Work out the finished part from the listing and answer in its coordinate system (mm). Give positions to 0.01 mm unless a question says otherwise; leave off trailing zeros. Loops run counter-clockwise (first coordinate to the right, second up) from the corner with the lowest first, then second, coordinate; pieces in that order, holes last. Notation, with made-up numbers: (24.25, 69.25) -> (48.25, 69.25) arc R28 ccw to (48.25, 95.25) -> close; hole circle Ø10 at (15, 78.25). An arc over 180 degrees is marked (long way). Answer as CSV lines item,"result". Start each with the question number.
1. Find the intervals of material crossed by line 1 along X through (y, z) = (70, 4.1); line 2 along X through (y, z) = (78, 1.3); line 3 along X through (y, z) = (6.5, 4.7), in increasing order.
2. Find section C-C, the plane x = 34. Give the vertices of the cut face in (y, z).
3. Determine the mould class of faces 1 (the face through (44.4, 87.7, 2.2)), 2 (the face through (77.5, 45, 3)), 3 (the face through (7.21, 9.73, 2.53)) for opening direction Y: +Y half, -Y half, draft (parallel to the pull), parting line (faces both ways), or undercut.
4. Find section D-D, the plane y = 51.5. Give the vertices of the cut face in (x, z), and give its area (3 significant figures).
5. Find section A-A, the plane x = 7.5. Give the vertices of the cut face in (y, z).
6. Flat-ended cylindrical pins translate along their axes: pin 1 Ø2 at (x, z) = (55, 2) entering from +Y; pin 2 Ø3 at (x, y) = (75, 12) entering from +Z; pin 3 Ø0.6 at (x, z) = (30, 1.5) entering from -Y. Find the tip coordinate at first contact, or state that the pin passes through.
7. Find section B-B, the plane y = 82.5. Give the vertices of the cut face in (x, z), and give its area (3 significant figures).
from build123d import *

# Parameters (mm, degrees)
SKETCH_W        = 90
SKETCH_H        = 90
PAD_DEPTH       = 5
SKETCH001_R     = 2.25
POCKET_DEPTH    = 5
SKETCH002_W     = 65
SKETCH002_H     = 71
POCKET001_DEPTH = 2
SKETCH003_R     = 0.9
POCKET002_DEPTH = 5
SKETCH004_W     = 65
SKETCH004_H     = 60
POCKET003_DEPTH = 3
CHAMFER_SIZE    = 4.5
CHAMFER001_SIZE = 1
CHAMFER002_SIZE = 0.5
CHAMFER003_SIZE = 0.5
CHAMFER004_SIZE = 0.5
CHAMFER005_SIZE = 0.5
CHAMFER006_SIZE = 1
CHAMFER007_SIZE = 0.5
CHAMFER008_SIZE = 0.5
CHAMFER009_SIZE = 0.4
CHAMFER010_SIZE = 0.5


with BuildPart() as part:
    # Sketch → Pad (new body)
    with BuildSketch(Plane.XY):
        with Locations((45, 45)):
            Rectangle(SKETCH_W, SKETCH_H)
    extrude(amount=PAD_DEPTH)

    # Sketch001 (on Face6 of Pad) → Pocket (cut)
    with BuildSketch(Plane.XY.offset(5)):
        with Locations((7.5, 82.5)):
            Circle(SKETCH001_R)
        with Locations((82.5, 82.5)):
            Circle(SKETCH001_R)
        with Locations((82.5, 7.5)):
            Circle(SKETCH001_R)
        with Locations((7.5, 7.5)):
            Circle(SKETCH001_R)
    extrude(amount=-POCKET_DEPTH, mode=Mode.SUBTRACT)

    # Sketch002 (on Face5 of Pocket) → Pocket001 (cut)
    with BuildSketch(Plane.XY.offset(5)):
        with Locations((45, 45)):
            Rectangle(SKETCH002_W, SKETCH002_H)
    extrude(amount=-POCKET001_DEPTH, mode=Mode.SUBTRACT)

    # Sketch003 (on Face15 of Pocket001) → Pocket002 (cut)
    with BuildSketch(Plane.XY.offset(3)):
        with Locations((15, 78)):
            Circle(SKETCH003_R)
        with Locations((41, 78)):
            Circle(SKETCH003_R)
        with Locations((41, 12)):
            Circle(SKETCH003_R)
        with Locations((15, 12)):
            Circle(SKETCH003_R)
        with Locations((49, 78)):
            Circle(SKETCH003_R)
        with Locations((75, 78)):
            Circle(SKETCH003_R)
        with Locations((75, 12)):
            Circle(SKETCH003_R)
        with Locations((49, 12)):
            Circle(SKETCH003_R)
    extrude(amount=-POCKET002_DEPTH, mode=Mode.SUBTRACT)

    # Sketch004 (on Face23 of Pocket002) → Pocket003 (cut)
    with BuildSketch(Plane.XY.offset(3)):
        with Locations((45, 45)):
            Rectangle(SKETCH004_W, SKETCH004_H)
    extrude(amount=-POCKET003_DEPTH, mode=Mode.SUBTRACT)

    # Chamfer
    chamfer_edges = [part.edges().sort_by_distance(p)[0] for p in [
        (45, 90, 0),
        (45, 0, 0),
    ]]
    chamfer(chamfer_edges, length=CHAMFER_SIZE)

    # Chamfer001
    chamfer001_edges = [part.edges().sort_by_distance(p)[0] for p in [
        (0, 45, 0),
        (90, 45, 0),
    ]]
    chamfer(chamfer001_edges, length=CHAMFER001_SIZE)

    # Chamfer002
    chamfer002_edges = [part.edges().sort_by_distance(p)[0] for p in [
        (45, 75, 0),
        (12.5, 45, 0),
        (45, 15, 0),
        (77.5, 45, 0),
    ]]
    chamfer(chamfer002_edges, length=CHAMFER002_SIZE)

    # Chamfer003
    chamfer003_edges = [part.edges().sort_by_distance(p)[0] for p in [
        (5.25, 7.5, 0),
        (80.25, 82.5, 0),
        (80.25, 7.5, 0),
        (5.25, 82.5, 0),
    ]]
    chamfer(chamfer003_edges, length=CHAMFER003_SIZE)

    # Chamfer004
    chamfer004_edges = [part.edges().sort_by_distance(p)[0] for p in [
        (14.1, 78, 0),
        (14.1, 12, 0),
        (40.1, 78, 0),
        (48.1, 12, 0),
        (40.1, 12, 0),
        (48.1, 78, 0),
        (74.1, 12, 0),
        (74.1, 78, 0),
    ]]
    chamfer(chamfer004_edges, length=CHAMFER004_SIZE)

    # Chamfer005
    chamfer005_edges = [part.edges().sort_by_distance(p)[0] for p in [
        (5.25, 7.5, 5),
        (80.25, 7.5, 5),
        (80.25, 82.5, 5),
        (5.25, 82.5, 5),
    ]]
    chamfer(chamfer005_edges, length=CHAMFER005_SIZE)

    # Chamfer006
    chamfer006_edges = [part.edges().sort_by_distance(p)[0] for p in [
        (74.1, 78, 3),
        (48.1, 78, 3),
        (14.1, 78, 3),
        (14.1, 12, 3),
        (40.1, 12, 3),
        (74.1, 12, 3),
        (48.1, 12, 3),
        (40.1, 78, 3),
    ]]
    chamfer(chamfer006_edges, length=CHAMFER006_SIZE)

    # Chamfer007
    chamfer007_edges = [part.edges().sort_by_distance(p)[0] for p in [
        (77.5, 45, 5),
        (45, 80.5, 5),
        (12.5, 45, 5),
        (45, 9.5, 5),
    ]]
    chamfer(chamfer007_edges, length=CHAMFER007_SIZE)

    # Chamfer008
    chamfer008_edges = [part.edges().sort_by_distance(p)[0] for p in [
        (45, 15, 3),
        (45, 75, 3),
    ]]
    chamfer(chamfer008_edges, length=CHAMFER008_SIZE)

    # Chamfer009
    chamfer009_edges = [part.edges().sort_by_distance(p)[0] for p in [
        (90, 45, 5),
        (45, 90, 5),
        (0, 45, 5),
        (45, 0, 5),
    ]]
    chamfer(chamfer009_edges, length=CHAMFER009_SIZE)

    # Chamfer010
    chamfer010_edges = [part.edges().sort_by_distance(p)[0] for p in [
        (90, 0, 4.55),
        (90, 90, 4.55),
        (0, 90, 4.55),
        (0, 0, 4.55),
    ]]
    chamfer(chamfer010_edges, length=CHAMFER010_SIZE)


solid = part.part
Resolved:
1,line 1,"x = 0 to 12.5, 77.5 to 90"
1,line 2,"x = 0 to 14.1, 15.9 to 40.1, 41.9 to 48.1, 49.9 to 74.1, 75.9 to 90"
1,line 3,"x = 0.1 to 5.26, 9.74 to 80.26, 84.74 to 89.9"
2,outline,"(0, 4.5) -> (4.5, 0) -> (14.5, 0) -> (15, 0.5) -> (15, 2.5) -> (14.5, 3) -> (9.5, 3) -> (9.5, 4.5) -> (9, 5) -> (0.4, 5) -> (0, 4.6) -> close; (75, 0.5) -> (75.5, 0) -> (85.5, 0) -> (90, 4.5) -> (90, 4.6) -> (89.6, 5) -> (81, 5) -> (80.5, 4.5) -> (80.5, 3) -> (75.5, 3) -> (75, 2.5) -> close"
3,face 1,"+Y half"
3,face 2,"undercut"
3,face 3,"undercut"
4,outline,"(0, 1) -> (1, 0) -> (12, 0) -> (12.5, 0.5) -> (12.5, 4.5) -> (12, 5) -> (0.4, 5) -> (0, 4.6) -> close; (77.5, 0.5) -> (78, 0) -> (89, 0) -> (90, 1) -> (90, 4.6) -> (89.6, 5) -> (78, 5) -> (77.5, 4.5) -> close"
4,area,"123 mm^2"
5,outline,"(0, 4.5) -> (4.5, 0) -> (4.75, 0) -> (5.25, 0.5) -> (5.25, 4.5) -> (4.75, 5) -> (0.4, 5) -> (0, 4.6) -> close; (9.75, 0.5) -> (10.25, 0) -> (79.75, 0) -> (80.25, 0.5) -> (80.25, 4.5) -> (79.75, 5) -> (10.25, 5) -> (9.75, 4.5) -> close; (84.75, 0.5) -> (85.25, 0) -> (85.5, 0) -> (90, 4.5) -> (90, 4.6) -> (89.6, 5) -> (85.25, 5) -> (84.75, 4.5) -> close"
6,pin 1,"stops at y = 88.5"
6,pin 2,"stops at z = 2.6"
6,pin 3,"stops at y = 2.7"
7,outline,"(0, 1) -> (1, 0) -> (4.75, 0) -> (5.25, 0.5) -> (5.25, 4.5) -> (4.75, 5) -> (0.4, 5) -> (0, 4.6) -> close; (9.75, 0.5) -> (10.25, 0) -> (79.75, 0) -> (80.25, 0.5) -> (80.25, 4.5) -> (79.75, 5) -> (10.25, 5) -> (9.75, 4.5) -> close; (84.75, 0.5) -> (85.25, 0) -> (89, 0) -> (90, 1) -> (90, 4.6) -> (89.6, 5) -> (85.25, 5) -> (84.75, 4.5) -> close"
7,area,"403 mm^2"
